Could you check a few things on this model? Use its own coordinates, in mm. A direction names the side the tool comes from. Give positions to 0.01 mm unless a question says otherwise; leave off trailing zeros. Loops run counter-clockwise (first coordinate to the right, second up) from the corner with the lowest first, then second, coordinate; pieces in that order, holes last. Notation, with made-up numbers: M 6,-7 L 60,-7 A30 ccw 60,31 Z; hole C 70.5,-2.5 d1. An arc over 180 degrees is marked long. Answer in a Markdown table with one row per item. Add a question column.
1. I'm going to push a flat-ended pin straight in: pin 1 Ø4.5 at (x, y) = (3.8, 3.8) entering from +Z. Where does the tip first touch, or does it pass through?
2. If we section it at A-A on x = 3.8: List the corners of the cut face in (y, z) for me, then the cut area to 3 significant figures.
3. Which directions (+Z, -Z, +X, -X, +Y, -Y) give clear straight access to the entire face, cutting with the end or side of a thin tool? Please do faces 4 (the flat face through (4, 6.8, 7)), 5 (the flat face through (0, 4, 4)).
4. Thinking about a two-plate mould opening in X: for faces 1 (the flat face through (7.6, 4, 4)), 2 (the flat face through (1.2, 5.3, 7)), 3 (the flat face through (1, 6, 8)), which applies, released by +X, released by -X, zero draft, split by the parting line, or undercut?
5. If we section it at D-D on y = 1.5: List the corners of the cut face in (x, z) for me.
6. If we section it at B-B on y = 3.5: List the corners of the cut face in (x, z) for me.
7. If we section it at C-C on z = 5.75: List the corners of the cut face in (x, y) for me, then the cut area to 3 significant figures.
8. I need wall thicknesses on line 1 along Y through (x, z) = (3.8, 3.35); line 2 along Y through (x, z) = (2.25, 7.75). Which ranges of each line are inside material? Lowest first, please. Write a range as from..to.
```python
from build123d import *

# Parameters (mm, degrees)
SKETCH1_W           = 7.6
SKETCH1_H           = 7.6
SKETCH1_R           = 1.7
BOSS_EXTRUDE1_DEPTH = 8
CUT_EXTRUDE1_DEPTH  = 2


with BuildPart() as part:
    # Sketch1 → Boss-Extrude1 (new body)
    with BuildSketch(Plane.XY):
        with Locations((3.8, 3.8)):
            Rectangle(SKETCH1_W, SKETCH1_H)
        with Locations((3.8, 3.8)):
            Circle(SKETCH1_R, mode=Mode.SUBTRACT)
    extrude(amount=BOSS_EXTRUDE1_DEPTH)

    # Sketch3 → Cut-Extrude1 (cut)
    with BuildSketch(Plane.XY.offset(8)):
        Polygon((5.532050808, 0.8), (7.264101615, 3.8), (5.532050808, 6.8), (2.067949192, 6.8), (0.335898385, 3.8), (2.067949192, 0.8), align=None)
    extrude(amount=-CUT_EXTRUDE1_DEPTH, mode=Mode.SUBTRACT)


solid = part.part
```
Results:
| question | item | result |
|---|---|---|
| 1 | pin 1 | z = 6 |
| 2 | outline | M 0,0 L 2.1,0 L 2.1,6 L 0.8,6 L 0.8,8 L 0,8 Z; M 5.5,0 L 7.6,0 L 7.6,8 L 6.8,8 L 6.8,6 L 5.5,6 Z |
| 2 | area | 28.4 mm2 |
| 3 | face 4 | +Z |
| 3 | face 5 | +Z, -Z, -X, +Y, -Y |
| 4 | face 1 | released by +X |
| 4 | face 2 | undercut |
| 4 | face 3 | zero draft |
| 5 | outline | M 0,0 L 7.6,0 L 7.6,8 L 5.94,8 L 5.94,6 L 1.66,6 L 1.66,8 L 0,8 Z |
| 6 | outline | M 0,0 L 2.13,0 L 2.13,6 L 0.51,6 L 0.51,8 L 0,8 Z; M 5.47,0 L 7.6,0 L 7.6,8 L 7.09,8 L 7.09,6 L 5.47,6 Z |
| 7 | outline | M 0,0 L 7.6,0 L 7.6,7.6 L 0,7.6 Z; hole C 3.8,3.8 d3.4 |
| 7 | area | 48.7 mm2 |
| 8 | line 1 | 0..2.1, 5.5..7.6 |
| 8 | line 2 | 0..0.8, 6.8..7.6 |
